from build123d import *

# Parameters (mm, degrees)
BOSS_EXTRUDE1_DEPTH = 18
SKETCH3_W           = 150
SKETCH3_H           = 140
CUT_EXTRUDE2_DEPTH  = 18
CUT_EXTRUDE3_DEPTH  = 18
SKETCH5_R           = 25
CUT_EXTRUDE4_DEPTH  = 1415.328109033


with BuildPart() as part:
    # Sketch1 → Boss-Extrude1 (new body)
    with BuildSketch(Plane(origin=(0, 0, 0), x_dir=(1, 0, 0), z_dir=(0, 1, 0))):
        Polygon((0, 0), (1000, 0), (1000, 430), (755, 430), (755, 1000), (0, 1000), align=None)
    extrude(amount=BOSS_EXTRUDE1_DEPTH)

    # Sketch3 → Cut-Extrude2 (cut)
    with BuildSketch(Plane(origin=(0, 18, 0), x_dir=(1, 0, 0), z_dir=(0, 1, 0))):
        with Locations((165, 160)):
            Rectangle(SKETCH3_W, SKETCH3_H)
    extrude(amount=-CUT_EXTRUDE2_DEPTH, mode=Mode.SUBTRACT)

    # Sketch4 → Cut-Extrude3 (cut)
    with BuildSketch(Plane(origin=(0, 18, 0), x_dir=(1, 0, 0), z_dir=(0, 1, 0))):
        Polygon((940, 60), (940, 175), (865, 175), (850, 190), (810, 190), (810, 150), (825, 135), (825, 60), align=None)
    extrude(amount=-CUT_EXTRUDE3_DEPTH, mode=Mode.SUBTRACT)

    # Sketch5 → Cut-Extrude4 (cut, through all)
    with BuildSketch(Plane(origin=(0, 18, 0), x_dir=(1, 0, 0), z_dir=(0, 1, 0))):
        with Locations(Location((500, 500, 0), (0, 0, 270))):
            Circle(SKETCH5_R)
    extrude(amount=-CUT_EXTRUDE4_DEPTH, mode=Mode.SUBTRACT)


solid = part.part
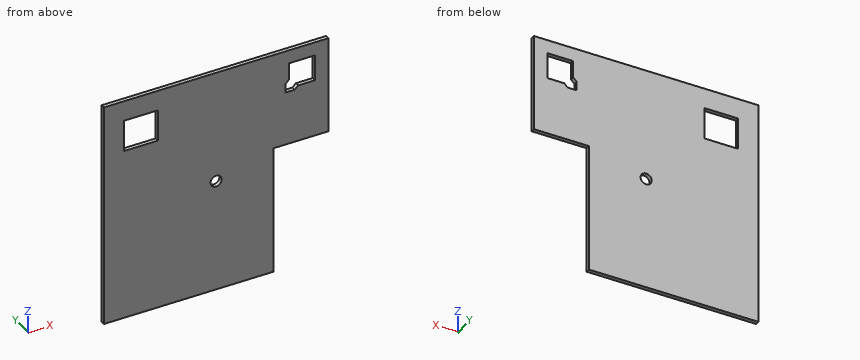
CAD build for the part. Positions are in the model's coordinates, mm. Round coordinates to 2 decimals unless told otherwise and drop trailing zeros. Loops run counter-clockwise (first coordinate to the right, second up) from the corner with the lowest first, then second, coordinate; pieces in that order, holes last.
(1) Cut at A-A (x = 500). Give the cut face in (y, z), plus the area to 3 significant figures.
(2) Cut at C-C (y = 5.25). Give the cut face in (x, z), plus the area to 3 significant figures.
(3) Cut at D-D (x = 796). Give the cut face in (y, z).
(4) Wall check: line 1 along X through (y, z) = (4.25, -97); line 2 along X through (y, z) = (11.25, -500); line 3 along X through (y, z) = (10.75, -156). Give the ranges that are in metal, low to high.
(5) Cut at B-B (z = -500). Give the cut face in (x, y).
(6) Drop a flat-ended pin along its axis: pin 1 (9 mm diameter, centred on x = 929.5, y = 12, fed in from -Z). Give the stop position or say it passes through.
Findings below:
1. outline: (0, -1000) - (18, -1000) - (18, -525) - (0, -525) - close; (0, -475) - (18, -475) - (18, 0) - (0, 0) - close
1. area: 17,100 mm2
2. outline: (0, -1000) - (755, -1000) - (755, -430) - (1000, -430) - (1000, 0) - (0, 0) - close; hole (90, -230) - (240, -230) - (240, -90) - (90, -90) - close; hole circle Ø50 at (500, -500); hole (810, -190) - (850, -190) - (865, -175) - (940, -175) - (940, -60) - (825, -60) - (825, -135) - (810, -150) - close
2. area: 823,000 mm2
3. outline: (0, -430) - (18, -430) - (18, 0) - (0, 0) - close
4. line 1: x = 0 to 90, 240 to 825, 940 to 1000
4. line 2: x = 0 to 475, 525 to 755
4. line 3: x = 0 to 90, 240 to 810, 940 to 1000
5. outline: (0, 0) - (475, 0) - (475, 18) - (0, 18) - close; (525, 0) - (755, 0) - (755, 18) - (525, 18) - close
6. pin 1: stops at z = -430
